from build123d import *

# Parameters (mm, degrees)
BOSS_EXTRUDE1_DEPTH = 25
BOSS_EXTRUDE3_REACH = 40.303


with BuildPart() as part:
    # Sketch2 → Boss-Extrude1 (new body)
    with BuildSketch(Plane(origin=(0, 0, 0), x_dir=(1, 0, 0), z_dir=(0, 1, 0))):
        Polygon((0, 0), (0, -15), (-5, -15), (-5, -2), (-9, -2), (-9, -15), (-14, -15), (-14, 5.798989873), align=None)
    boss_extrude1 = extrude(amount=BOSS_EXTRUDE1_DEPTH)

    # Mirror1: Boss-Extrude1 across plane
    add(boss_extrude1.mirror(Plane(origin=(0, 25, 0), x_dir=(0.9238795325112891, 0, 0.382683432365084), z_dir=(-0.382683432365084, 0, 0.9238795325112892))))

    # Boss-Extrude3: up to this plane
    boss_extrude3_end = Plane(origin=(10.606601718, 25, -10.606601718), z_dir=(0.7071067811865388, 0, -0.7071067811865563))
    # Sketch4 → Boss-Extrude3 (add, up to the surface)
    with BuildSketch(Plane(origin=(0, 0, 0), x_dir=(-0.9238795325112892, 0, -0.38268343236508406), z_dir=(0.3826834323650841, 0, -0.9238795325112893)), mode=Mode.PRIVATE) as boss_extrude3_sk1:
        Polygon((0, 0), (-5, -8.660254038), (10.153490804, -8.660254038), (15.153490804, 0), align=None)
    boss_extrude3_tool1 = split(extrude(boss_extrude3_sk1.sketch, amount=BOSS_EXTRUDE3_REACH, dir=(0.707106781187, 0, -0.707106781187), mode=Mode.PRIVATE), bisect_by=boss_extrude3_end, keep=Keep.BOTH, mode=Mode.PRIVATE)
    add(boss_extrude3_tool1.solids().sort_by_distance((-4.690301, -4.330127, -1.942786))[0])


solid = part.part
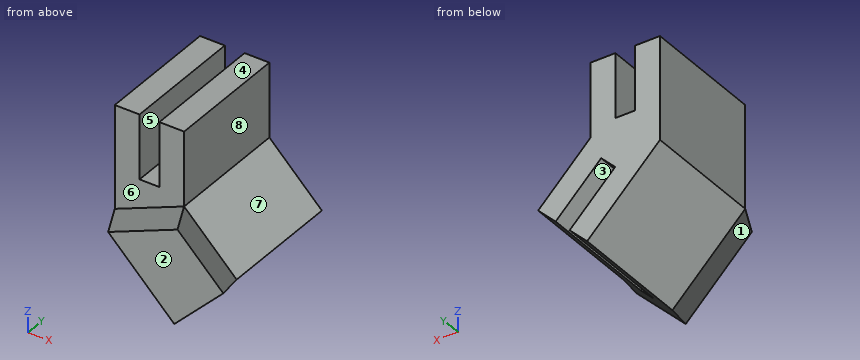
Can you work these out from the model? Positions are in its coordinate system, mm. Face numbers are marked on the shaded views. A direction names the side the tool comes from. Round coordinates to 2 decimals unless told otherwise and drop trailing zeros. Order: outer loops, then holes, each group sorted by start corner. A loop starts at its lowest first (then second) coordinate and runs counter-clockwise, first axis right, second up. Notation, with made-up numbers: M -28.5,85 L 24.5,85 A21 ccw 24.5,109 Z; hole C 77.25,69 d11. An arc over 180 degrees is marked long. Use a Markdown table: item, result.
1) If I drill on line 1 along X through (y, z) = (1.5, 8); line 2 along Y through (x, z) = (-1.5, 8); line 3 along Z through (x, y) = (4, 8.5), over which ranges is the centre line in solid material (lowest first)?
Geometry says:
| item | result |
|---|---|
| line 1 | x = -14 to -9, -5 to 0 |
| line 2 | y = 0 to 25 |
| line 3 | z = -17.21 to -16.73, -11.07 to -4 |
2) On a 3-axis mill with a long thin cutter (end or side, diameter ignored), from which of +Z, -Z, +X, -X, +Y, -Y can I reach the whole of each face in a straight line? I mean the marked faces 5, 6, 7 and 8. Say none if no direction works.
Geometry says:
| item | result |
|---|---|
| face 5 | +Z, +Y, -Y |
| face 6 | +Z, -X, -Y |
| face 7 | +Z, +X, +Y |
| face 8 | +Z, +X, +Y, -Y |
3) If we mould it in two halves opening along Z, with no side actions, what happens to the marked faces 1, 2, 3 and 4? For each: +Z half, -Z half, draft (parallel to the pull), parting line (faces both ways), or undercut.
Geometry says:
| item | result |
|---|---|
| face 1 | -Z half |
| face 2 | draft |
| face 3 | undercut |
| face 4 | +Z half |
4) Imagine slicing it at C-C (x = -5.5). List the corners of the cut face in (y, z) for me.
Geometry says:
| item | result |
|---|---|
| outline | M -8.66,-7.77 L 0,-14.3 L 25,-14.3 L 25,2 L 0,2 L 0,-2.28 L -8.66,-2.28 Z |
5) I'm going to push flat-ended pins straight in: P1, Ø1.5, axis at x = 2.5, y = 0.5, coming from the -Z side; P2, Ø6, axis at y = 2, z = -12.5, coming from the -X side; P3, Ø3, axis at x = 8.5, y = 5, coming from the -Z side. Where does each tip first touch, or does it pass through?
Geometry says:
| item | result |
|---|---|
| P1 | stops at z = -19.46 |
| P2 | stops at x = -10.3 |
| P3 | stops at z = -14.14 |
6) Imagine slicing it at A-A (z = 3.5). List the corners of the cut face in (x, y) for me, then the cut area to 3 significant figures.
Geometry says:
| item | result |
|---|---|
| outline | M -14,0 L -9,0 L -9,25 L -14,25 Z; M -5,0 L 0,0 L 0,25 L -5,25 Z |
| area | 250 mm² |
7) Imagine slicing it at D-D (z = -9). List the corners of the cut face in (x, y) for me.
Geometry says:
| item | result |
|---|---|
| outline | M -10.8,0 L -4.27,-8.66 L 12.21,-8.66 L 12.21,-4.26 L 9,0 L 9,25 L 1.93,25 L 1.93,0 L -3.73,0 L -3.73,25 L -10.8,25 Z |
8) Imagine slicing it at B-B (y = 3). List the corners of the cut face in (x, z) for me, then the cut area to 3 significant figures.
Geometry says:
| item | result |
|---|---|
| outline | M -14,-5.8 L 0.71,-20.51 L 4.24,-16.97 L -4.95,-7.78 L -2.12,-4.95 L 7.07,-14.14 L 10.61,-10.61 L 0,0 L 0,15 L -5,15 L -5,2 L -9,2 L -9,15 L -14,15 Z |
| area | 397 mm² |
